Build history of the part. All positions in model axes, mm. Face numbers are marked on the shaded views. A direction names the side the tool comes from. Round coordinates to 2 decimals unless told otherwise and drop trailing zeros. Write each loop counter-clockwise with the first axis right and the second up, starting at its lowest first coordinate (ties: lowest second). Pieces come first, ordered by that corner, then holes. Notation, with made-up numbers: (54, 74) -> (110, 74) arc R23 cw to (110, 87) -> close; hole circle Ø5 at (62.5, 65). An arc over 180 degrees is marked (long way). Answer in a Markdown table with one row per item.
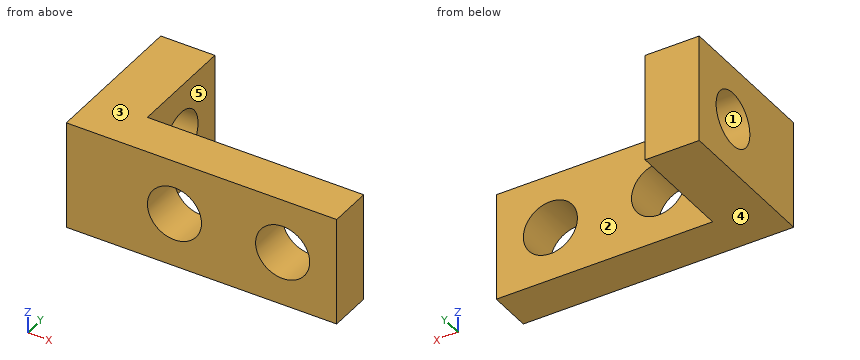
```python
from build123d import *

# Parameters (mm, degrees)
SKETCH1_W           = 12.7
SKETCH1_H           = 6.35
SKETCH1_R           = 1.5875
BOSS_EXTRUDE1_DEPTH = 2.54
SKETCH2_W           = 6.35
SKETCH2_H           = 8.89
SKETCH2_R           = 1.5875
BOSS_EXTRUDE2_DEPTH = 3.175


with BuildPart() as part:
    # Sketch1 → Boss-Extrude1 (new body)
    with BuildSketch(Plane(origin=(0, 0, 0), x_dir=(1, 0, 0), z_dir=(0, 1, 0))):
        with Locations((-6.35, 3.175)):
            Rectangle(SKETCH1_W, SKETCH1_H)
        with Locations((-3.175, 3.175)):
            Circle(SKETCH1_R, mode=Mode.SUBTRACT)
        with Locations((-9.525, 3.175)):
            Circle(SKETCH1_R, mode=Mode.SUBTRACT)
    extrude(amount=BOSS_EXTRUDE1_DEPTH)

    # Sketch2 → Boss-Extrude2 (add)
    with BuildSketch(Plane.ZY.offset(12.7)):
        with Locations((-3.175, 4.445)):
            Rectangle(SKETCH2_W, SKETCH2_H)
        with Locations((-3.175, 5.715)):
            Circle(SKETCH2_R, mode=Mode.SUBTRACT)
    extrude(amount=BOSS_EXTRUDE2_DEPTH)


solid = part.part
```
Q1. Saw through at C-C on z = -4.5. Write the cut outline in (x, y) (3 decimals).
A:
| item | result |
|---|---|
| outline | (-15.875, 0) -> (-10.399, 0) -> (-10.399, 2.54) -> (-12.7, 2.54) -> (-12.7, 4.841) -> (-15.875, 4.841) -> close; (-15.875, 6.589) -> (-12.7, 6.589) -> (-12.7, 8.89) -> (-15.875, 8.89) -> close; (-8.651, 0) -> (-4.049, 0) -> (-4.049, 2.54) -> (-8.651, 2.54) -> close; (-2.301, 0) -> (0, 0) -> (0, 2.54) -> (-2.301, 2.54) -> close |
Q2. Wall check: line 1 (Y direction, x = -12, z = -1.25); line 2 (X direction, y = 4.75, z = -5.75) (3 decimals); line 3 (Z direction, x = -2.25, y = 2). Give the ranges that are in metal, low to high. Write a range as [from, to].
A:
| item | result |
|---|---|
| line 1 | [0, 2.54] |
| line 2 | [-15.875, -12.7] |
| line 3 | [-6.35, -4.47], [-1.88, 0] |
Q3. Drop flat-ended pins along their axis: P1, Ø3, axis at y = 5.715, z = -3.175, coming from the -X side; P2, Ø3.5, axis at x = -3.175, z = -3.175, coming from the +Y side; P3, Ø1.9, axis at y = 6, z = -2, coming from the +X side. Give the stop position or say it passes through.
A:
| item | result |
|---|---|
| P1 | through |
| P2 | y = 2.54 |
| P3 | x = -12.7 |
Q4. Two-plate mould, pull along Y, no slides. Class the marked faces 1, 2 and 3: released by +Y, released by -Y, zero draft, split by the parting line, or undercut.
A:
| item | result |
|---|---|
| face 1 | undercut |
| face 2 | released by +Y |
| face 3 | zero draft |
Q5. Which spindle directions (+Z, -Z, +X, -X, +Y, -Y) get a long thin tool onto all of the face, cutting with end or side? Do the marked faces 4 and 5. Say none if no direction does.
A:
| item | result |
|---|---|
| face 4 | -Z, +X, -X, +Y, -Y |
| face 5 | +Z, -Z, +X, +Y |
Q6. Saw through at B-B on y = 5. Write the cut outline in (x, z) (3 decimals), plus the area to 3 significant figures.
A:
| item | result |
|---|---|
| outline | (-15.875, -6.35) -> (-12.7, -6.35) -> (-12.7, -4.592) -> (-15.875, -4.592) -> close; (-15.875, -1.758) -> (-12.7, -1.758) -> (-12.7, 0) -> (-15.875, 0) -> close |
| area | 11.2 mm² |
Q7. Saw through at A-A on x = -3.5. Write the cut outline in (y, z), plus the area to 3 significant figures.
A:
| item | result |
|---|---|
| outline | (0, -6.35) -> (2.54, -6.35) -> (2.54, -4.73) -> (0, -4.73) -> close; (0, -1.62) -> (2.54, -1.62) -> (2.54, 0) -> (0, 0) -> close |
| area | 8.24 mm² |
